Could you check a few things on this model? Use its own coordinates, in mm. A direction names the side the tool comes from. Give positions to 0.01 mm unless a question says otherwise; leave off trailing zeros. Order: outer loops, then holes, each group sorted by start corner. A loop starts at its lowest first (then second) coordinate and runs counter-clockwise, first axis right, second up. Notation, with made-up numbers: (58, 23.5) - (108, 23.5) arc R22 cw to (108, 40.5) - close; hole circle Ø11 at (-32, -28). An arc over 180 degrees is marked (long way). One line per question, with ' | ' between items. Start each with the question number.
1. Imagine slicing it at D-D (y = -1). Please give me the cut outline in (x, z) (3 decimals).
2. Which directions (+Z, -Z, +X, -X, +Y, -Y) give clear straight access to the entire face, cutting with the end or side of a thin tool? Please do faces 1 (the flat face through (0, 15, -7)), 2 (the flat face through (0, -10.65, 0)), 3 (the cylindrical face through (5.56, -15.171, 2.385)), 4 (the flat face through (0, -15, -9)).
3. Imagine slicing it at B-B (y = 12.5). Please give me the cut outline in (x, z) (3 decimals).
4. If we mould it in two halves opening along Z, with no side actions, what happens to faces 5 (the cylindrical face through (-1.187, -12.129, -1.547)), 6 (the flat face through (0, 10.65, 0)), 7 (the cylindrical face through (17.72, -0.19, -5.14)), 8 (the cylindrical face through (6.038, -15.171, 0.707))? For each: released by +Z, released by -Z, zero draft, split by the parting line, or undercut.
5. For P1, Ø0.9, axis at y = 15.5, z = -7, coming from the -X side; P2, Ø1.7, axis at x = 49.5, y = 6, coming from the +Z side; P3, Ø4, axis at x = 26.5, y = -4.5, coming from the +Z side; P4, Ø1.5, axis at x = 42.5, z = -4, coming from the -Y side, each with a flat end and sliding along its axis, tell me the tip position at first contact or that it passes through.
6. Imagine slicing it at A-A (x = 11). Please give me the cut outline in (y, z).
7. Imagine slicing it at C-C (z = 2.5). Please give me the cut outline in (x, y), and give its area (3 significant figures).
8. I need wall thicknesses on probe 1 along Y at (x, z) = (8.5, -3.5); probe 2 along X at (y, z) = (-14.5, -5); probe 3 along X at (y, z) = (-1.5, -3). Which ranges of each line are inside material? Lowest first, please. Write a range as from..to.
```python
from build123d import *

# Parameters (mm, degrees)
SKETCH1_W           = 50
SKETCH1_H           = 10
BOSS_EXTRUDE2_DEPTH = 16.65
CUT_EXTRUDE1_START  = -27.3
SKETCH2_R           = 18.45
CUT_EXTRUDE1_DEPTH  = 27.3
SKETCH3_R           = 4
BOSS_EXTRUDE3_DEPTH = 3
BOSS_EXTRUDE4_START = 3
SKETCH5_R           = 4
BOSS_EXTRUDE4_DEPTH = 3
SKETCH4_R           = 1.95
BOSS_EXTRUDE6_DEPTH = 3
BOSS_EXTRUDE5_START = 3
SKETCH6_R           = 1.95
BOSS_EXTRUDE5_DEPTH = 3
BOSS_EXTRUDE7_DEPTH = 3
SKETCH8_R           = 15
CUT_EXTRUDE2_DEPTH  = 61.900656811
FILLET1_R           = 15


with BuildPart() as part:
    # Sketch1 → Boss-Extrude2 (new, symmetric)
    with BuildSketch(Plane(origin=(0, 0, 0), x_dir=(1, 0, 0), z_dir=(0, 1, 0))):
        with Locations((25, 5)):
            Rectangle(SKETCH1_W, SKETCH1_H)
    extrude(amount=BOSS_EXTRUDE2_DEPTH, both=True)

    # Sketch2 → Cut-Extrude1 (cut)
    with BuildSketch(Plane(origin=(0, 13.65, 0), x_dir=(1, 0, 0), z_dir=(0, 1, 0)).offset(CUT_EXTRUDE1_START)):
        Circle(SKETCH2_R)
    extrude(amount=CUT_EXTRUDE1_DEPTH, mode=Mode.SUBTRACT)

    # Sketch3 → Boss-Extrude3 (add)
    with BuildSketch(Plane(origin=(0, 13.65, 0), x_dir=(1, 0, 0), z_dir=(0, 1, 0))):
        Circle(SKETCH3_R)
    extrude(amount=BOSS_EXTRUDE3_DEPTH)

    # Sketch5 → Boss-Extrude4 (add)
    with BuildSketch(Plane(origin=(0, -13.65, 0), x_dir=(-1, 0, 0), z_dir=(0, -1, 0)).offset(BOSS_EXTRUDE4_START)):
        Circle(SKETCH5_R)
    extrude(amount=-BOSS_EXTRUDE4_DEPTH)

    # Sketch4 → Boss-Extrude6 (add)
    with BuildSketch(Plane.XZ.offset(-13.65)):
        with Locations(Location((0, 0, 0), (0, 0, 90))):
            Circle(SKETCH4_R)
    extrude(amount=BOSS_EXTRUDE6_DEPTH)

    # Sketch6 → Boss-Extrude5 (add)
    with BuildSketch(Plane(origin=(0, -13.65, 0), x_dir=(1, 0, 0), z_dir=(0, 1, 0)).offset(BOSS_EXTRUDE5_START)):
        with Locations(Location((0, 0, 0), (0, 0, 270))):
            Circle(SKETCH6_R)
    extrude(amount=-BOSS_EXTRUDE5_DEPTH)

    # Sketch7 → Boss-Extrude7 (add)
    with BuildSketch(Plane.XZ.offset(16.65)):
        with BuildLine():
            ThreePointArc((1.103045949, -4.464319525), (1.190197866, -4.441878907), (1.276893949, -4.417737093))
            ThreePointArc((1.276893949, -4.417737093), (1.56039667, -4.439315905), (1.760385559, -4.6414146))
            ThreePointArc((1.760385559, -4.6414146), (2.395683629, -5.570836958), (3.313490513, -6.222803277))
            ThreePointArc((3.313490513, -6.222803277), (3.525, -6.105479097), (3.732360464, -5.980968598))
            ThreePointArc((3.732360464, -5.980968598), (3.626644512, -4.860141361), (3.139390174, -3.845245915))
            ThreePointArc((3.139390174, -3.845245915), (3.064362014, -3.571001109), (3.187425576, -3.314691145))
            ThreePointArc((3.187425576, -3.314691145), (3.251681041, -3.251681041), (3.314691145, -3.187425576))
            ThreePointArc((3.314691145, -3.187425576), (3.571001109, -3.064362014), (3.845245915, -3.139390174))
            ThreePointArc((3.845245915, -3.139390174), (4.860141361, -3.626644512), (5.980968598, -3.732360464))
            ThreePointArc((5.980968598, -3.732360464), (6.105479097, -3.525), (6.222803277, -3.313490513))
            ThreePointArc((6.222803277, -3.313490513), (5.570836958, -2.395683629), (4.6414146, -1.760385559))
            ThreePointArc((4.6414146, -1.760385559), (4.439315905, -1.56039667), (4.417737093, -1.276893949))
            ThreePointArc((4.417737093, -1.276893949), (4.441878907, -1.190197866), (4.464319525, -1.103045949))
            ThreePointArc((4.464319525, -1.103045949), (4.624758685, -0.868314796), (4.899775733, -0.796168685))
            ThreePointArc((4.899775733, -0.796168685), (6.022328141, -0.710695597), (7.045850977, -0.241834679))
            ThreePointArc((7.045850977, -0.241834679), (7.05, 0), (7.045850977, 0.241834679))
            ThreePointArc((7.045850977, 0.241834679), (6.022328141, 0.710695597), (4.899775733, 0.796168685))
            ThreePointArc((4.899775733, 0.796168685), (4.624758685, 0.868314796), (4.464319525, 1.103045949))
            ThreePointArc((4.464319525, 1.103045949), (4.441878907, 1.190197866), (4.417737093, 1.276893949))
            ThreePointArc((4.417737093, 1.276893949), (4.439315905, 1.56039667), (4.6414146, 1.760385559))
            ThreePointArc((4.6414146, 1.760385559), (5.570836958, 2.395683629), (6.222803277, 3.313490513))
            ThreePointArc((6.222803277, 3.313490513), (6.105479097, 3.525), (5.980968598, 3.732360464))
            ThreePointArc((5.980968598, 3.732360464), (4.860141361, 3.626644512), (3.845245915, 3.139390174))
            ThreePointArc((3.845245915, 3.139390174), (3.571001109, 3.064362014), (3.314691145, 3.187425576))
            ThreePointArc((3.314691145, 3.187425576), (3.251681041, 3.251681041), (3.187425576, 3.314691145))
            ThreePointArc((3.187425576, 3.314691145), (3.064362014, 3.571001109), (3.139390174, 3.845245915))
            ThreePointArc((3.139390174, 3.845245915), (3.626644512, 4.860141361), (3.732360464, 5.980968598))
            ThreePointArc((3.732360464, 5.980968598), (3.525, 6.105479097), (3.313490513, 6.222803277))
            ThreePointArc((3.313490513, 6.222803277), (2.395683629, 5.570836958), (1.760385559, 4.6414146))
            ThreePointArc((1.760385559, 4.6414146), (1.56039667, 4.439315905), (1.276893949, 4.417737093))
            ThreePointArc((1.276893949, 4.417737093), (1.190197866, 4.441878907), (1.103045949, 4.464319525))
            ThreePointArc((1.103045949, 4.464319525), (0.868314796, 4.624758685), (0.796168685, 4.899775733))
            ThreePointArc((0.796168685, 4.899775733), (0.710695597, 6.022328141), (0.241834679, 7.045850977))
            ThreePointArc((0.241834679, 7.045850977), (0, 7.05), (-0.241834679, 7.045850977))
            ThreePointArc((-0.241834679, 7.045850977), (-0.710695597, 6.022328141), (-0.796168685, 4.899775733))
            ThreePointArc((-0.796168685, 4.899775733), (-0.868314796, 4.624758685), (-1.103045949, 4.464319525))
            ThreePointArc((-1.103045949, 4.464319525), (-1.190197866, 4.441878907), (-1.276893949, 4.417737093))
            ThreePointArc((-1.276893949, 4.417737093), (-1.56039667, 4.439315905), (-1.760385559, 4.6414146))
            ThreePointArc((-1.760385559, 4.6414146), (-2.395683629, 5.570836958), (-3.313490513, 6.222803277))
            ThreePointArc((-3.313490513, 6.222803277), (-3.525, 6.105479097), (-3.732360464, 5.980968598))
            ThreePointArc((-3.732360464, 5.980968598), (-3.626644512, 4.860141361), (-3.139390174, 3.845245915))
            ThreePointArc((-3.139390174, 3.845245915), (-3.064362014, 3.571001109), (-3.187425576, 3.314691145))
            ThreePointArc((-3.187425576, 3.314691145), (-3.251681041, 3.251681041), (-3.314691145, 3.187425576))
            ThreePointArc((-3.314691145, 3.187425576), (-3.571001109, 3.064362014), (-3.845245915, 3.139390174))
            ThreePointArc((-3.845245915, 3.139390174), (-4.860141361, 3.626644512), (-5.980968598, 3.732360464))
            ThreePointArc((-5.980968598, 3.732360464), (-6.105479097, 3.525), (-6.222803277, 3.313490513))
            ThreePointArc((-6.222803277, 3.313490513), (-5.570836958, 2.395683629), (-4.6414146, 1.760385559))
            ThreePointArc((-4.6414146, 1.760385559), (-4.439315905, 1.56039667), (-4.417737093, 1.276893949))
            ThreePointArc((-4.417737093, 1.276893949), (-4.441878907, 1.190197866), (-4.464319525, 1.103045949))
            ThreePointArc((-4.464319525, 1.103045949), (-4.624758685, 0.868314796), (-4.899775733, 0.796168685))
            ThreePointArc((-4.899775733, 0.796168685), (-6.022328141, 0.710695597), (-7.045850977, 0.241834679))
            ThreePointArc((-7.045850977, 0.241834679), (-7.05, 0), (-7.045850977, -0.241834679))
            ThreePointArc((-7.045850977, -0.241834679), (-6.022328141, -0.710695597), (-4.899775733, -0.796168685))
            ThreePointArc((-4.899775733, -0.796168685), (-4.624758685, -0.868314796), (-4.464319525, -1.103045949))
            ThreePointArc((-4.464319525, -1.103045949), (-4.441878907, -1.190197866), (-4.417737093, -1.276893949))
            ThreePointArc((-4.417737093, -1.276893949), (-4.439315905, -1.56039667), (-4.6414146, -1.760385559))
            ThreePointArc((-4.6414146, -1.760385559), (-5.570836958, -2.395683629), (-6.222803277, -3.313490513))
            ThreePointArc((-6.222803277, -3.313490513), (-6.105479097, -3.525), (-5.980968598, -3.732360464))
            ThreePointArc((-5.980968598, -3.732360464), (-4.860141361, -3.626644512), (-3.845245915, -3.139390174))
            ThreePointArc((-3.845245915, -3.139390174), (-3.571001109, -3.064362014), (-3.314691145, -3.187425576))
            ThreePointArc((-3.314691145, -3.187425576), (-3.251681041, -3.251681041), (-3.187425576, -3.314691145))
            ThreePointArc((-3.187425576, -3.314691145), (-3.064362014, -3.571001109), (-3.139390174, -3.845245915))
            ThreePointArc((-3.139390174, -3.845245915), (-3.626644512, -4.860141361), (-3.732360464, -5.980968598))
            ThreePointArc((-3.732360464, -5.980968598), (-3.525, -6.105479097), (-3.313490513, -6.222803277))
            ThreePointArc((-3.313490513, -6.222803277), (-2.395683629, -5.570836958), (-1.760385559, -4.6414146))
            ThreePointArc((-1.760385559, -4.6414146), (-1.56039667, -4.439315905), (-1.276893949, -4.417737093))
            ThreePointArc((-1.276893949, -4.417737093), (-1.190197866, -4.441878907), (-1.103045949, -4.464319525))
            ThreePointArc((-1.103045949, -4.464319525), (-0.868314796, -4.624758685), (-0.796168685, -4.899775733))
            ThreePointArc((-0.796168685, -4.899775733), (-0.710695597, -6.022328141), (-0.241834679, -7.045850977))
            ThreePointArc((-0.241834679, -7.045850977), (0, -7.05), (0.241834679, -7.045850977))
            ThreePointArc((0.241834679, -7.045850977), (0.710695597, -6.022328141), (0.796168685, -4.899775733))
            ThreePointArc((0.796168685, -4.899775733), (0.868314796, -4.624758685), (1.103045949, -4.464319525))
        make_face()
    extrude(amount=-BOSS_EXTRUDE7_DEPTH)

    # Sketch8 → Cut-Extrude2 (cut, through all)
    with BuildSketch(Plane.XZ.offset(16.65)):
        with Locations((34.225, 6.15)):
            Circle(SKETCH8_R)
    extrude(amount=-CUT_EXTRUDE2_DEPTH, mode=Mode.SUBTRACT)

    # Fillet1
    # the kernel refuses this fillet: 15 mm, written as the material it takes off along each edge
    with BuildSketch(Plane(origin=(50, -52.005339059, -10), x_dir=(-1, 0, 0), z_dir=(0, 1, 0))) as fillet1_piece_1:
        with BuildLine():
            CenterArc((14.142135624, 15), FILLET1_R, 199.471220634, 70.528779366)
            Line((0, 10), (-0.282842712, 9.9))
            ThreePointArc((-0.282842712, 9.9), (-0.3, 5), (-0.3, 0))
            Line((-0.3, 0), (0, -0.3))
            Line((0, -0.3), (14.142135624, -0.3))
            Line((14.142135624, -0.3), (14.142135624, 0))
        make_face()
    extrude(amount=104.010678119, mode=Mode.SUBTRACT)


solid = part.part
```
Results found:
1) outline: (15.505, -10) - (35.858, -10) arc R15 ccw to (50, 0) - (47.906, 0) arc R15 cw to (20.544, 0) - (18.45, 0) arc R18.45 cw to start
2) face 1: -Z, -X, +Y | face 2: +Z, -Z, -X | face 3: +X, +Y, -Y | face 4: -Z, -X, +Y, -Y
3) outline: circle Ø3.9 at (0, 0); (15.505, -10) - (35.858, -10) arc R15 ccw to (50, 0) - (47.906, 0) arc R15 cw to (20.544, 0) - (18.45, 0) arc R18.45 cw to start
4) face 5: split by the parting line | face 6: zero draft | face 7: released by +Z | face 8: undercut
5) P1: stops at x = 0 | P2: stops at z = 0 | P3: stops at z = -5.27 | P4: passes through
6) outline: (-16.65, -10) - (-13.65, -10) - (-13.65, 0) - (-16.65, 0) - close; (13.65, -10) - (16.65, -10) - (16.65, 0) - (13.65, 0) - close
7) outline: (-5.67, -16.65) - (5.67, -16.65) - (5.67, -13.65) - (-5.67, -13.65) - close; (-3.12, 13.65) - (3.12, 13.65) - (3.12, 16.65) - (-3.12, 16.65) - close | area: 52.8 mm2
8) probe 1: y = -16.65..-13.65, 13.65..16.65 | probe 2: x = -3.66..-1.95, -0.8..24.19, 44.26..47.04 | probe 3: x = 18.2..22.34, 46.11..48.55
